Geometry: final body of the model. Coordinates: model frame, mm. Face numbers are marked on the shaded views. A direction names the side the tool comes from. Give positions to 0.01 mm unless a question says otherwise; leave off trailing zeros. Loops run counter-clockwise (first coordinate to the right, second up) from the corner with the lowest first, then second, coordinate; pieces in that order, holes last. Notation, with made-up numbers: (-24.5, 78.25) - (26.5, 78.25) arc R13 ccw to (26.5, 100.25) - close; hole circle Ø5 at (73.25, 16.5). An arc over 180 degrees is marked (long way). Answer in a Markdown table with one row per item.
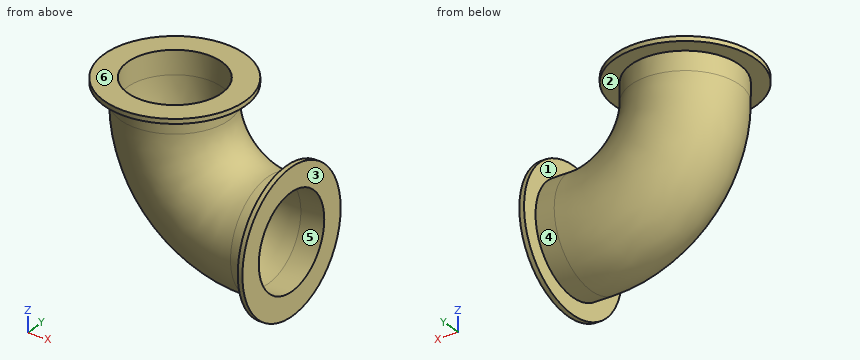
from build123d import *

# Parameters (mm, degrees)
F2_R     = 29.21
F2_R_2   = 25.4
F4_R     = 38.1
F4_R_2   = 25.4
F5_DEPTH = 2.54
F6_R     = 38.1
F6_R_2   = 25.4
F7_DEPTH = 2.54


with BuildPart() as f3:
    # F3: sweep along a path in F0
    with BuildLine(Plane.XZ) as f3_path:
        Line((12.7, 0), (0, 0))
        ThreePointArc((0, 0), (-35.921024, 14.878976), (-50.8, 50.8))
        Line((-50.8, 50.8), (-50.8, 63.5))
    # F2 (on offset) → F3 (sweep)
    with BuildSketch(Plane.YZ.offset(12.7)):
        Circle(F2_R)
        Circle(F2_R_2, mode=Mode.SUBTRACT)
    sweep(path=f3_path.line)

    # F4 (on face) → F5 (join)
    with BuildSketch(Plane.YZ.offset(12.7)):
        Circle(F4_R)
        Circle(F4_R_2, mode=Mode.SUBTRACT)
    extrude(amount=-F5_DEPTH)

    # F6 (on face) → F7 (join)
    with BuildSketch(Plane.XY.offset(63.5)):
        with Locations((-50.8, 0)):
            Circle(F6_R)
        with Locations((-50.8, 0)):
            Circle(F6_R_2, mode=Mode.SUBTRACT)
    extrude(amount=-F7_DEPTH)


solid = f3.part
Q1. Cut plane B-B (x = -19). Give the number of separate pieces and of enclosed holes in the cut face, and give its area (3 significant figures).
Check values:
| item | result |
|---|---|
| separate pieces | 2 |
| enclosed holes | 1 |
| area | 881 mm² |
Q2. Material intervals for line 1 along Z through (x, y) = (3, 0); line 2 along X through (y, z) = (-10, 41), sorted ascending.
Check values:
| item | result |
|---|---|
| line 1 | -29.21 to -25.4, 25.4 to 29.21 |
| line 2 | -77.63 to -73.5, -25.64 to -21.2 |
Q3. Draft query along X for the marked faces 1, 2 and 3. Return one class per face: pulls with the +X half, pulls with the -X half, needs draft (parallel to the pull), parting line crosses it, or undercut.
Check values:
| item | result |
|---|---|
| face 1 | undercut |
| face 2 | needs draft |
| face 3 | pulls with the +X half |
Q4. Reachability of the marked faces 4, 5 and 6 from +Z, -Z, +X, -X, +Y, -Y: full face, straight path, thin tool, end or side. Return the list, or none.
Check values:
| item | result |
|---|---|
| face 4 | none |
| face 5 | +X |
| face 6 | +Z, +X, -X, +Y, -Y |
Q5. Cut plane A-A (x = 4). Output: boundary loops of the cut face in (y, z), and give its area (3 significant figures).
Check values:
| item | result |
|---|---|
| outline | circle Ø58.42 at (0, 0); hole circle Ø50.8 at (0, 0) |
| area | 654 mm² |
Q6. First-contact query: pin 1 (2 mm diameter, centred on x = -25, y = 14, fed in from -Z); pin 2 (1 mm diameter, centred on x = -67.5, z = 36.5, fed in from +Y); pin 3 (2 mm diameter, centred on y = 25, z = -19.5, fed in from -X). Flat tips, straight axial feed; report the tip coordinate or a pass-through.
Check values:
| item | result |
|---|---|
| pin 1 | z = -22.08 |
| pin 2 | y = 23.24 |
| pin 3 | x = 10.16 |
